Autodesk Inventor part; units mm, degrees
ref_plane "YZ Plane" through (0, 0, 0) normal (1, 0, 0) x (0, 1, 0)
ref_plane "XZ Plane" through (0, 0, 0) normal (0, 1, 0) x (-1, 0, 0)
ref_plane "XY Plane" through (0, 0, 0) normal (0, 0, 1) x (1, 0, 0)
sketch "Sketch2" plane through (0, 0, 0) normal (0, 0, 1) x (1, 0, 0)
  line L0 (-15, 0) -> (15, 0)
  line L1 (15, 0) -> (15, 2.5)
  line L2 (15, 2.5) -> (-15, 2.5)
  line L3 (-15, 2.5) -> (-15, 0)
  line L4 (15, 2.5) -> (10, 2.5)
  line L5 (10, 2.5) -> (10, 1.5)
  line L6 (10, 1.5) -> (15, 1.5)
  line L7 (15, 1.5) -> (15, 2.5)
  line L8 (-15, 2.5) -> (-10, 2.5)
  line L9 (-10, 2.5) -> (-10, 1.5)
  line L10 (-10, 1.5) -> (-15, 1.5)
  line L11 (-15, 1.5) -> (-15, 2.5)
  point P0 (0, 0)
  point P1 (0, 0)
  dimension "d3" = 30
  dimension "d4" = 2.5
  dimension "d5" = 1.5
  dimension "d6" = 5
revolve "Revolution1" add sketch "Sketch2" angle 360 about axis through (-15, 0, 0) along (1, 0, 0) contours L3 L10 L9 L2 L5 L6 L1 L0
properties part number "Pin" material "Stainless Steel"
CAD build for the part. Positions are in the model's coordinates, mm. A direction names the side the tool comes from. Give positions to 0.01 mm unless a question says otherwise; leave off trailing zeros. Loops run counter-clockwise (first coordinate to the right, second up) from the corner with the lowest first, then second, coordinate; pieces in that order, holes last. Notation, with made-up numbers: M 50.25,39.5 L 76.25,39.5 A17 cw 76.25,51.5 Z; hole C 77.25,-17.5 d5. An arc over 180 degrees is marked long. One line per question, with ' | ' between items. Start each with the question number.
1. Saw through at A-A on y = 0. Give the cut face in (x, z).
2. Flat gauge pin, fed straight in: pin 1 (2 mm diameter, centred on x = 11.5, z = 1.5, fed in from -Y). Where does the tip first touch, or does it go through?
3. Probe L1, parallel to X at y = 1, z = 1.4; L2, parallel to Z at x = 10.75, y = -0.7; L3, parallel to Z at x = 9.5, y = 0.9. List the from-to ranges inside material, lowest first. Write a range as from..to.
4. Saw through at D-D on y = 2.1. Give the cut face in (x, z), plus the area to 3 significant figures.
5. 3-axis set-ups, long thin cutter, end or side, ignore diameter. For faces 1 (the face through (15, 0, 0)), 2 (the face through (10, 2, 0)), 3 (the face through (-10, 2, 0)): which of +Z, -Z, +X, -X, +Y, -Y reach the whole face in a straight line?
6. Saw through at C-C on x = 1.25. Give the cut face in (y, z), plus the area to 3 significant figures.
Result sheet:
1) outline: M -15,-1.5 L -10,-1.5 L -10,-2.5 L 10,-2.5 L 10,-1.5 L 15,-1.5 L 15,1.5 L 10,1.5 L 10,2.5 L -10,2.5 L -10,1.5 L -15,1.5 Z
2) pin 1: stops at y = -1.41
3) L1: x = -10..10 | L2: z = -1.33..1.33 | L3: z = -2.33..2.33
4) outline: M -10,-1.36 L 10,-1.36 L 10,1.36 L -10,1.36 Z | area: 54.3 mm^2
5) face 1: +Z, -Z, +X, +Y, -Y | face 2: +X | face 3: -X
6) outline: C 0,0 d5 | area: 19.6 mm^2
